from build123d import *

# Parameters (mm, degrees)
CHAMFER1_SIZE = 0.25
CHAMFER3_SIZE = 0.5
CHAMFER4_SIZE = 0.25
FILLET1_R     = 0.25


with BuildPart() as part:
    # Sketch1 → Revolve1 (revolve)
    with BuildSketch(Plane.XY, mode=Mode.PRIVATE) as revolve1_sk:
        Polygon((-1, 4.2), (-3, 4.2), (-3, 1), (-2, 0), (-3, -1), (-3, -4), (-2, -4), (-2, -8), (-3, -8), (-3, -12), (-2, -12), (-2, -13), (-1, -13), align=None)
    revolve(revolve1_sk.sketch.rotate(Axis((0, 54.199953661, 0), (0, -1, 0)), 270), axis=Axis((0, 54.199953661, 0), (0, -1, 0)))

    # Chamfer1
    chamfer1_edges = [part.edges().sort_by_distance(p)[0] for p in [
        (0, 4.2, -1),
    ]]
    chamfer(chamfer1_edges, length=CHAMFER1_SIZE)

    # Chamfer3
    chamfer3_edges = [part.edges().sort_by_distance(p)[0] for p in [
        (0, -13, -2),
    ]]
    chamfer(chamfer3_edges, length=CHAMFER3_SIZE)

    # Chamfer4
    chamfer4_edges = [part.edges().sort_by_distance(p)[0] for p in [
        (0, -4, -3),
        (0, 4.2, -3),
    ]]
    chamfer(chamfer4_edges, length=CHAMFER4_SIZE)

    # Fillet1
    fillet1_edges = [part.edges().sort_by_distance(p)[0] for p in [
        (0, 0, -2),
    ]]
    fillet(fillet1_edges, radius=FILLET1_R)


solid = part.part
Source: CAD feature listing. Evaluate the final solid. Frame: model axes, mm. A direction names the side the tool comes from. Give positions to 0.01 mm unless a question says otherwise; leave off trailing zeros. Write each loop counter-clockwise with the first axis right and the second up, starting at its lowest first coordinate (ties: lowest second). Pieces come first, ordered by that corner, then holes. Notation, with made-up numbers: (-16, -14.5) -> (-3, -14.5) arc R32 ccw to (-3, 14.5) -> close; hole circle Ø7 at (77, 11). An arc over 180 degrees is marked (long way). Return JSON: item names as keys, results as strings. Group by question number.
1. Section A-A, the plane y = -10. Output: boundary loops of the cut face in (x, z).
2. Mould query, pull axis Z, two halves, no side actions, for faces 4 (the face through (2, -12, 1)), 5 (the face through (-0.9, 2.45, 2.86)), 6 (the face through (1, -4, 0)). Classes: +Z half, -Z half, draft (parallel to the pull), parting line (faces both ways), or undercut.
3. Section B-B, the plane y = -5.5. Output: boundary loops of the cut face in (x, z).
4. Pin query (flat end, axial travel): pin 1 Ø3 at (x, y) = (-2.5, -11) entering from +Z; pin 2 Ø1.5 at (x, y) = (1, -9.5) entering from +Z; pin 3 Ø1.5 at (y, z) = (2.5, -0.5) entering from +X; pin 4 Ø1.5 at (y, z) = (-10, 1.5) entering from +X. Return the tip coordinate at first contact, or that it passes through.
5. Access query for faces 1 (the face through (1.952, -12.253, -0.434)), 2 (the face through (-0.9, -10.03, 2.86)), 3 (the face through (2, -8, -1)). Directions: +Z, -Z, +X, -X, +Y, -Y. A direction counts if a zero-diameter tool reaches every point of the face in a straight line with its end or side. Return the directions, or none.
6. Material intervals for line 1 (X direction, y = 0.75, z = 0); line 2 (X direction, y = -9, z = 0); line 3 (Y direction, x = 1.75, z = -2.25), sorted ascending. Write a range as from..to.
Determined:
{
 "1": {"outline": "circle Ø6 at (0, 0); hole circle Ø2 at (0, 0)"},
 "2": {"face 4": "draft", "face 5": "parting line", "face 6": "undercut"},
 "3": {"outline": "circle Ø4 at (0, 0); hole circle Ø2 at (0, 0)"},
 "4": {"pin 1": "stops at z = 2.83", "pin 2": "stops at z = 2.99", "pin 3": "stops at x = 3", "pin 4": "stops at x = 2.9"},
 "5": {"face 1": "-Y", "face 2": "+Y, -Y", "face 3": "none"},
 "6": {"line 1": "x = -2.75..-1, 1..2.75", "line 2": "x = -3..-1, 1..3", "line 3": "y = -12..-8, -3.9..-0.85, 0.85..4.1"}
}
